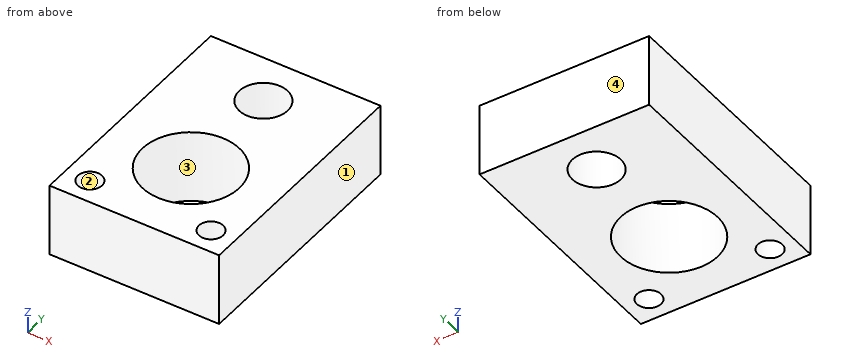
Autodesk Inventor part; units mm, degrees
ref_plane "YZ Plane" through (0, 0, 0) normal (1, 0, 0) x (0, 1, 0)
ref_plane "XZ Plane" through (0, 0, 0) normal (0, 1, 0) x (-1, 0, 0)
ref_plane "XY Plane" through (0, 0, 0) normal (0, 0, 1) x (1, 0, 0)
sketch "Sketch1" plane through (0, 0, 0) normal (0, 0, 1) x (1, 0, 0)
  line L0 (0, 0) -> (8.89, 0)
  line L1 (8.89, 0) -> (8.89, 12.7)
  line L2 (8.89, 12.7) -> (0, 12.7)
  line L3 (0, 12.7) -> (0, 0)
  dimension "d0" = 8.89
  dimension "d1" = 12.7
extrude "Extrusion1" add sketch "Sketch1" along normal blind 3.81
sketch "Sketch2" plane through (0, 0, 3.81) normal (0, 0, 1) x (1, 0, 0)
  circle A0 centre (4.4501, 4.445) radius 3.175
  line L0 (0, 0) -> (8.89, 0)
  line L1 (8.89, 0) -> (8.89, 12.7)
  dimension "d4" = 6.35
  dimension "d5" = 4.445
  dimension "d6" = 4.4399
hole "Hole1" at (4.4501, 4.445, 3.81) direction (0, 0, -1) diameter 5.08 depth 19.05
sketch "Sketch3" plane through (0, 0, 3.81) normal (0, 0, 1) x (1, 0, 0)
  circle A0 centre (4.445, 10.16) radius 1.27
  line L0 (8.89, 12.7) -> (0, 12.7)
  line L1 (8.89, 0) -> (8.89, 12.7)
  point P0 (0, 0)
  dimension "d14" = 2.54
  dimension "d15" = 2.54
  dimension "d16" = 4.445
extrude "Extrusion2" cut sketch "Sketch3" against normal blind 25.4
sketch "Sketch4" plane through (0, 0, 3.81) normal (0, 0, 1) x (1, 0, 0)
  circle A0 centre (7.62, 1.27) radius 0.635
  circle A1 centre (1.27, 1.27) radius 0.635
  line L0 (8.89, 0) -> (8.89, 12.7)
  line L1 (0, 0) -> (8.89, 0)
  line L2 (0, 12.7) -> (0, 0)
  dimension "d19" = 1.27
  dimension "d20" = 1.27
  dimension "d21" = 1.27
  dimension "d22" = 1.27
  dimension "d23" = 1.27
  dimension "d24" = 1.27
extrude "Extrusion3" cut sketch "Sketch4" against normal through all
properties part number "EndHole"
Verification items for the finished model (mm, model axes). Face numbers are marked on the shaded views. Coordinates: 2 decimals unless noted, no trailing zeros. Write each loop counter-clockwise with the first axis right and the second up, starting at its lowest first coordinate (ties: lowest second). Pieces come first, ordered by that corner, then holes. Notation, with made-up numbers: M -32.75,-24 L -22.75,-24 A13 ccw -22.75,-20 Z; hole C 34.25,10.5 d10. An arc over 180 degrees is marked long. Use a Markdown table: item, result.
Q1. Sectioned sample at A-A, the plane y = 1.27. Record the boundary of the cut face in (x, z) (3 decimals), plus the area to 3 significant figures.
Reply:
| item | result |
|---|---|
| outline | M 0,0 L 0.635,0 L 0.635,3.81 L 0,3.81 Z; M 1.905,0 L 6.985,0 L 6.985,3.81 L 1.905,3.81 Z; M 8.255,0 L 8.89,0 L 8.89,3.81 L 8.255,3.81 Z |
| area | 24.2 mm² |
Q2. Draft check along Y on the marked faces 1, 2, 3 and 4. Enter one of: +Y half, -Y half, draft (parallel to the pull), parting line (faces both ways), or undercut.
Reply:
| item | result |
|---|---|
| face 1 | draft |
| face 2 | undercut |
| face 3 | undercut |
| face 4 | +Y half |
Q3. Go/stop test with a flat-tipped pin: P1, Ø1.1, axis at x = 7.62, y = 1.27, coming from the +Z side. Record where the tip stops, or that it passes through.
Reply:
| item | result |
|---|---|
| P1 | passes through |
Q4. Sectioned sample at D-D, the plane z = 0.7. Record the boundary of the cut face in (x, y) (3 decimals).
Reply:
| item | result |
|---|---|
| outline | M 0,0 L 8.89,0 L 8.89,12.7 L 0,12.7 Z; hole C 1.27,1.27 d1.27; hole C 4.45,4.445 d5.08; hole C 4.445,10.16 d2.54; hole C 7.62,1.27 d1.27 |
Q5. Sectioned sample at C-C, the plane y = 10.16. Record the boundary of the cut face in (x, z) (3 decimals).
Reply:
| item | result |
|---|---|
| outline | M 0,0 L 3.175,0 L 3.175,3.81 L 0,3.81 Z; M 5.715,0 L 8.89,0 L 8.89,3.81 L 5.715,3.81 Z |
Q6. Thickness scan on line 1 (Y direction, x = 5, z = 2.3); line 2 (Y direction, x = 5.5, z = 0.3); line 3 (X direction, y = 1.5, z = 1.6). Record the ranges inside material, lowest first.
Reply:
| item | result |
|---|---|
| line 1 | y = 0 to 1.97, 6.92 to 9.02, 11.3 to 12.7 |
| line 2 | y = 0 to 2.13, 6.76 to 9.45, 10.87 to 12.7 |
| line 3 | x = 0 to 0.68, 1.86 to 7.03, 8.21 to 8.89 |
Q7. Sectioned sample at B-B, the plane x = 7.62. Record the boundary of the cut face in (y, z) (3 decimals).
Reply:
| item | result |
|---|---|
| outline | M 0,0 L 0.635,0 L 0.635,3.81 L 0,3.81 Z; M 1.905,0 L 12.7,0 L 12.7,3.81 L 1.905,3.81 Z |
